Could you check a few things on this model? Use its own coordinates, in mm. A direction names the side the tool comes from. Round coordinates to 2 decimals unless told otherwise and drop trailing zeros. Write each loop counter-clockwise with the first axis right and the second up, starting at its lowest first coordinate (ties: lowest second). Pieces come first, ordered by that corner, then holes. Notation, with made-up numbers: (-36.75, 11) -> (-7.75, 11) arc R22 ccw to (-7.75, 32) -> close; hole circle Ø8 at (-33.75, 9). An arc over 180 degrees is marked (long way). Return JSON: item names as keys, results as strings.
from build123d import *

# Parameters (mm, degrees)
BOSS_EXTRUDE1_START = 1
SKETCH1_R           = 32.5
SKETCH1_R_2         = 21
BOSS_EXTRUDE1_DEPTH = 1
SKETCH2_R           = 32.5
BOSS_EXTRUDE2_DEPTH = 8
SKETCH3_R           = 2.5
CUT_EXTRUDE1_DEPTH  = 47.834816109


with BuildPart() as part:
    # Sketch1 → Boss-Extrude1 (new body)
    with BuildSketch(Plane.XY.offset(BOSS_EXTRUDE1_START)):
        Circle(SKETCH1_R)
        Circle(SKETCH1_R_2, mode=Mode.SUBTRACT)
    extrude(amount=BOSS_EXTRUDE1_DEPTH)

    # Sketch2 → Boss-Extrude2 (add)
    with BuildSketch(Plane.XY.offset(2)):
        Circle(SKETCH2_R)
    extrude(amount=BOSS_EXTRUDE2_DEPTH)

    # Sketch3 → Cut-Extrude1 (cut, through all)
    with BuildSketch(Plane.XY.offset(10)):
        with Locations((0, 27.783091373)):
            Circle(SKETCH3_R)
        with Locations((27.783091373, 0)):
            Circle(SKETCH3_R)
        with Locations((0, -27.783091373)):
            Circle(SKETCH3_R)
        with Locations((-27.783091373, 0)):
            Circle(SKETCH3_R)
    extrude(amount=-CUT_EXTRUDE1_DEPTH, mode=Mode.SUBTRACT)


solid = part.part
1) I want a section at D-D, the plane z = 4.5. Please give me the cut outline in (x, y).
Return value:
{"outline": "circle Ø65 at (0, 0); hole circle Ø5 at (-27.78, 0); hole circle Ø5 at (0, -27.78); hole circle Ø5 at (0, 27.78); hole circle Ø5 at (27.78, 0)"}
2) I want a section at A-A, the plane x = 0. Please give me the cut outline in (y, z).
Return value:
{"outline": "(-32.5, 1) -> (-30.28, 1) -> (-30.28, 10) -> (-32.5, 10) -> close; (-25.28, 1) -> (-21, 1) -> (-21, 2) -> (21, 2) -> (21, 1) -> (25.28, 1) -> (25.28, 10) -> (-25.28, 10) -> close; (30.28, 1) -> (32.5, 1) -> (32.5, 10) -> (30.28, 10) -> close"}
3) For faces 1 (the face through (21.2, 0.5, 1)), 2 (the face through (20.03, 6.31, 1.49)), which set-ups out of +Z, -Z, +X, -X, +Y, -Y let a thin tool reach every point of the face, with its end or its side?
Return value:
{"face 1": "-Z, +X, -X, +Y, -Y", "face 2": "-Z"}
4) Will these pins go through, and if not, where does the flat tip stop? pin 1 Ø5 at (x, z) = (-9.5, 5.5) entering from -Y; pin 2 Ø21 at (x, y) = (-0.5, -9.5) entering from -Z; pin 3 Ø1.5 at (y, z) = (21, 9) entering from +X.
Return value:
{"pin 1": "y = -31.74", "pin 2": "z = 2", "pin 3": "x = 25.42"}
5) Thinking about a two-plate mould opening in Y: for faces 3 (the face through (-0.33, 30.26, 5.56)), 4 (the face through (31, 9.76, 5.44)), 5 (the face through (0, 0, 10)), which applies, pulls with the +Y half, pulls with the -Y half, needs draft (parallel to the pull), parting line crosses it, or undercut?
Return value:
{"face 3": "undercut", "face 4": "parting line crosses it", "face 5": "needs draft"}
6) If I drill on probe 1 along Y at (x, z) = (0, 1.65); probe 2 along X at (y, z) = (-1, 8.5); probe 3 along Y at (x, z) = (26.5, 2), over which ranges is the centre line in solid material (lowest first)? Write a range as [from, to].
Return value:
{"probe 1": "[-32.5, -30.28], [-25.28, -21], [21, 25.28], [30.28, 32.5]", "probe 2": "[-32.48, -30.07], [-25.49, 25.49], [30.07, 32.48]", "probe 3": "[-18.81, -2.15], [2.15, 18.81]"}
7) I want a section at C-C, the plane x = 28. Please give me the cut outline in (y, z), and give its area (3 significant figures).
Return value:
{"outline": "(-16.5, 1) -> (-2.49, 1) -> (-2.49, 10) -> (-16.5, 10) -> close; (2.49, 1) -> (16.5, 1) -> (16.5, 10) -> (2.49, 10) -> close", "area": "252 mm²"}
